```python
from build123d import *

# Parameters (mm, degrees)
SKETCH_W     = 165
SKETCH_H     = 225
PAD_DEPTH    = 5
SKETCH001_W  = 150.1
SKETCH001_H  = 200.2
POCKET_DEPTH = 3
FILLET_R     = 3


with BuildPart() as part:
    # Sketch (on XY_Plane001 of Origin002) → Pad (new body)
    with BuildSketch(Plane.XY):
        Rectangle(SKETCH_W, SKETCH_H)
    extrude(amount=PAD_DEPTH)

    # Sketch001 (on Face6 of Pad) → Pocket (cut)
    with BuildSketch(Plane.XY.offset(5)):
        with Locations((7.45, 0)):
            Rectangle(SKETCH001_W, SKETCH001_H)
    extrude(amount=-POCKET_DEPTH, mode=Mode.SUBTRACT)

    # Fillet
    fillet_edges = [part.edges().sort_by_distance(p)[0] for p in [
        (-82.5, 112.5, 2.5),
        (-82.5, -112.5, 2.5),
    ]]
    fillet(fillet_edges, radius=FILLET_R)


solid = part.part
```
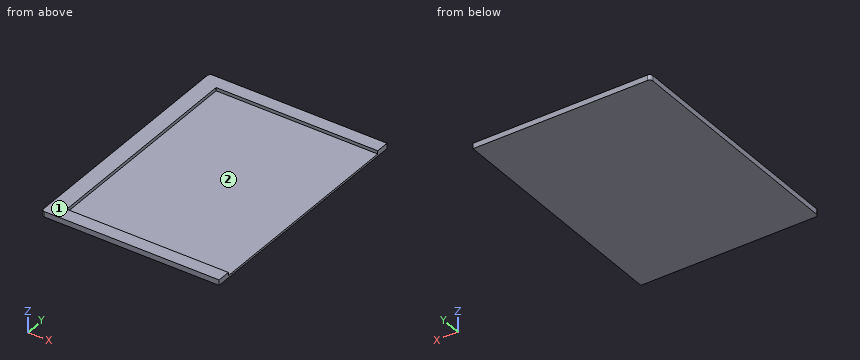
Here's how the part is built. I have some questions about the finished solid (model axes, mm). Face numbers are marked on the shaded views. Give positions to 0.01 mm unless a question says otherwise; leave off trailing zeros. Loops run counter-clockwise (first coordinate to the right, second up) from the corner with the lowest first, then second, coordinate; pieces in that order, holes last. Notation, with made-up numbers: M 21.5,30.5 L 29.5,30.5 A8 cw 29.5,42.5 Z; hole C -27.5,-12.5 d3. An arc over 180 degrees is marked long. Put each result on its own line as item: value. Start each with the question number.
(1) I need wall thicknesses on line 1 along Y through (x, z) = (45, 2.45); line 2 along Z through (x, y) = (36, 9); line 3 along X through (y, z) = (-93, 4.3). Which ranges of each line are inside material? Lowest first, please. Write a range as [from, to].
(2) I want a section at A-A on z = 4.15. Please give me the cut outline in (x, y), then the cut area to 3 significant figures.
(3) I want a section at C-C on y = -1. Please give me the cut outline in (x, z), then the cut area to 3 significant figures.
(4) I want a section at B-B on x = -54. Please give me the cut outline in (y, z), then the cut area to 3 significant figures.
(5) If we mould it in two halves opening along Y, with no side actions, what happens to the marked faces 1 and 2? For each: +Y half, -Y half, draft (parallel to the pull), parting line (faces both ways), or undercut.
(6) Will these pins go through, and if not, where does the flat tip stop? pin 1 Ø10 at (x, y) = (7.5, 30.5) entering from +Z; pin 2 Ø1.5 at (y, z) = (-11.5, 4) entering from +X.
Answer block:
1. line 1: [-112.5, -100.1], [100.1, 112.5]
1. line 2: [0, 2]
1. line 3: [-82.5, -67.6]
2. outline: M -82.5,-109.5 A3 ccw -79.5,-112.5 L 82.5,-112.5 L 82.5,-100.1 L -67.6,-100.1 L -67.6,100.1 L 82.5,100.1 L 82.5,112.5 L -79.5,112.5 A3 ccw -82.5,109.5 Z
2. area: 7,070 mm^2
3. outline: M -82.5,0 L 82.5,0 L 82.5,2 L -67.6,2 L -67.6,5 L -82.5,5 Z
3. area: 375 mm^2
4. outline: M -112.5,0 L 112.5,0 L 112.5,5 L 100.1,5 L 100.1,2 L -100.1,2 L -100.1,5 L -112.5,5 Z
4. area: 524 mm^2
5. face 1: draft
5. face 2: undercut
6. pin 1: z = 2
6. pin 2: x = -67.6
